Input: part model. Units: mm. Frame: model coordinates. A direction names the side the tool comes from. Round coordinates to 2 decimals unless told otherwise and drop trailing zeros. Write each loop counter-clockwise with the first axis right and the second up, starting at its lowest first coordinate (ties: lowest second). Pieces come first, ordered by that corner, then holes. Notation, with made-up numbers: (53.5, 28.5) -> (69.5, 28.5) arc R35 ccw to (69.5, 63.5) -> close; hole circle Ø10 at (82.5, -25.5). An arc over 180 degrees is marked (long way). Write item = value, one per line.
```python
from build123d import *

# Parameters (mm, degrees)
F1_DEPTH = 6
F3_DEPTH = 8


with BuildPart() as f1:
    # F0 (on Front) → F1 (new body)
    with BuildSketch(Plane.XZ):
        with BuildLine():
            ThreePointArc((7.8698224852, 39.1124260355), (2.0444516128, 30.3346375712), (0, 20))
            Line((0, 20), (10, 20))
            Line((10, 20), (10, 34))
            ThreePointArc((10, 34), (7.2307692308, 35.8461538462), (7.8698224852, 39.1124260355))
        make_face()
        with BuildLine():
            Line((10, 34), (10, 20))
            Line((10, 20), (20, 20))
            ThreePointArc((20, 20), (17.9555483872, 30.3346375712), (12.1301775148, 39.1124260355))
            ThreePointArc((12.1301775148, 39.1124260355), (12.7740342954, 38.1422494158), (13, 37))
            ThreePointArc((13, 37), (12.1213203436, 34.8786796564), (10, 34))
        make_face()
        with BuildLine():
            Line((10, 20), (0, 20))
            ThreePointArc((0, 20), (2.0444516128, 9.6653624288), (7.8698224852, 0.8875739645))
            ThreePointArc((7.8698224852, 0.8875739645), (7.2307692308, 4.1538461538), (10, 6))
            Line((10, 6), (10, 20))
        make_face()
        with BuildLine():
            Line((10, 20), (10, 6))
            ThreePointArc((10, 6), (12.1213203436, 5.1213203436), (13, 3))
            ThreePointArc((13, 3), (12.7740342954, 1.8577505842), (12.1301775148, 0.8875739645))
            ThreePointArc((12.1301775148, 0.8875739645), (17.9555483872, 9.6653624288), (20, 20))
            Line((20, 20), (10, 20))
        make_face()
        with BuildLine():
            ThreePointArc((7.8698224852, 0.8875739645), (8.8461538462, 0.2307692308), (10, 0))
            Line((10, 0), (10, 6))
            ThreePointArc((10, 6), (7.2307692308, 4.1538461538), (7.8698224852, 0.8875739645))
        make_face()
        with BuildLine():
            Line((10, 6), (10, 0))
            ThreePointArc((10, 0), (11.1538461538, 0.2307692308), (12.1301775148, 0.8875739645))
            ThreePointArc((12.1301775148, 0.8875739645), (12.7740342954, 1.8577505842), (13, 3))
            ThreePointArc((13, 3), (12.1213203436, 5.1213203436), (10, 6))
        make_face()
        with BuildLine():
            ThreePointArc((10, 40), (8.8461538462, 39.7692307692), (7.8698224852, 39.1124260355))
            ThreePointArc((7.8698224852, 39.1124260355), (7.2307692308, 35.8461538462), (10, 34))
            Line((10, 34), (10, 40))
        make_face()
        with BuildLine():
            ThreePointArc((12.1301775148, 39.1124260355), (11.1538461538, 39.7692307692), (10, 40))
            Line((10, 40), (10, 34))
            ThreePointArc((10, 34), (12.1213203436, 34.8786796564), (13, 37))
            ThreePointArc((13, 37), (12.7740342954, 38.1422494158), (12.1301775148, 39.1124260355))
        make_face()
    extrude(amount=F1_DEPTH)

    # F2 (on face) → F3 (join)
    with BuildSketch(Plane.XZ.offset(6)):
        with BuildLine():
            ThreePointArc((8.9349112426, 1.9437869822), (10, 1.5), (11.0650887574, 1.9437869822))
            ThreePointArc((11.0650887574, 1.9437869822), (16.5685312395, 10.2364871367), (18.5, 20))
            Line((18.5, 20), (2.4724225514, 20))
            Line((2.4724225514, 20), (1.5, 20))
            ThreePointArc((1.5, 20), (3.4314687605, 10.2364871367), (8.9349112426, 1.9437869822))
        make_face()
        with BuildLine():
            Line((2.4724225514, 20), (18.5, 20))
            ThreePointArc((18.5, 20), (16.5685312395, 29.7635128633), (11.0650887574, 38.0562130178))
            ThreePointArc((11.0650887574, 38.0562130178), (10, 38.5), (8.9349112426, 38.0562130178))
            ThreePointArc((8.9349112426, 38.0562130178), (3.4314687605, 29.7635128633), (1.5, 20))
            Line((1.5, 20), (2.4724225514, 20))
        make_face()
        with BuildLine():
            ThreePointArc((18.5, 20), (16.5685312395, 10.2364871367), (11.0650887574, 1.9437869822))
            ThreePointArc((11.0650887574, 1.9437869822), (16.9287608071, 10.1385897944), (19, 20))
            Line((19, 20), (18.5, 20))
        make_face()
        with BuildLine():
            ThreePointArc((11.0650887574, 38.0562130178), (16.5685312395, 29.7635128633), (18.5, 20))
            Line((18.5, 20), (19, 20))
            ThreePointArc((19, 20), (16.9287608071, 29.8614102056), (11.0650887574, 38.0562130178))
        make_face()
        with BuildLine():
            ThreePointArc((1, 20), (3.0712391929, 10.1385897944), (8.9349112426, 1.9437869822))
            ThreePointArc((8.9349112426, 1.9437869822), (3.4314687605, 10.2364871367), (1.5, 20))
            Line((1.5, 20), (1, 20))
        make_face()
        with BuildLine():
            Line((1, 20), (1.5, 20))
            ThreePointArc((1.5, 20), (3.4314687605, 29.7635128633), (8.9349112426, 38.0562130178))
            ThreePointArc((8.9349112426, 38.0562130178), (3.0712391929, 29.8614102056), (1, 20))
        make_face()
    extrude(amount=F3_DEPTH)


solid = f1.part
```
1) Cut plane B-B (z = 21.5). Return the cut outline in (x, y), and give its area (3 significant figures).
Solutions:
outline = (0.04, -6) -> (1.05, -6) -> (1.05, -14) -> (18.95, -14) -> (18.95, -6) -> (19.96, -6) -> (19.96, 0) -> (0.04, 0) -> close
area = 263 mm^2
2) Cut plane C-C (x = 17). Return the cut outline in (y, z).
Solutions:
outline = (-14, 10.3) -> (-6, 10.3) -> (-6, 7.6) -> (0, 7.6) -> (0, 32.4) -> (-6, 32.4) -> (-6, 29.7) -> (-14, 29.7) -> close
3) Access query for faces 1 (the face through (10, -9.9, 38.5)), 2 (the face through (1, -6, 23)), 3 (the face through (10, -9.9, 1.5)), 4 (the face through (10, 0, 20)), 5 (the face through (10, -14, 20)). Directions: +Z, -Z, +X, -X, +Y, -Y. A direction counts if a zero-diameter tool reaches every point of the face in a straight line with its end or side. Return the directions, or none.
Solutions:
face_1 = +Z, -Y
face_2 = -Y
face_3 = -Z, -Y
face_4 = +Z, -Z, +X, -X, +Y
face_5 = +Z, -Z, +X, -X, -Y
4) First-contact query: P1, Ø6, axis at y = -8.5, z = 25, coming from the -X side; P2, Ø3, axis at x = 17.5, y = -6, coming from the -Z side; P3, Ø5, axis at x = 14.5, y = -11.5, coming from the +Z side. Flat tips, straight axial feed; report the tip coordinate or a pass-through.
Solutions:
P1 = 0.21
P2 = 5.82
P3 = 37.15
5) Line query: L1, parallel to X at y = -7.75, z = 20; L2, parallel to X at y = -1.5, z = 20.5; L3, parallel to Z at x = 4, y = -2.75. Output: solid intervals per line, ascending. Write a range as from..to.
Solutions:
L1 = 1..19
L2 = 0..20
L3 = 5.82..34.18
6) Cut plane A-A (y = -6.75). Return the cut outline in (x, z).
Solutions:
outline = (8.93, 1.94) arc R1.5 ccw to (11.07, 1.94) arc R24.51 ccw to (11.07, 38.06) arc R1.5 ccw to (8.93, 38.06) arc R24.51 ccw to start
